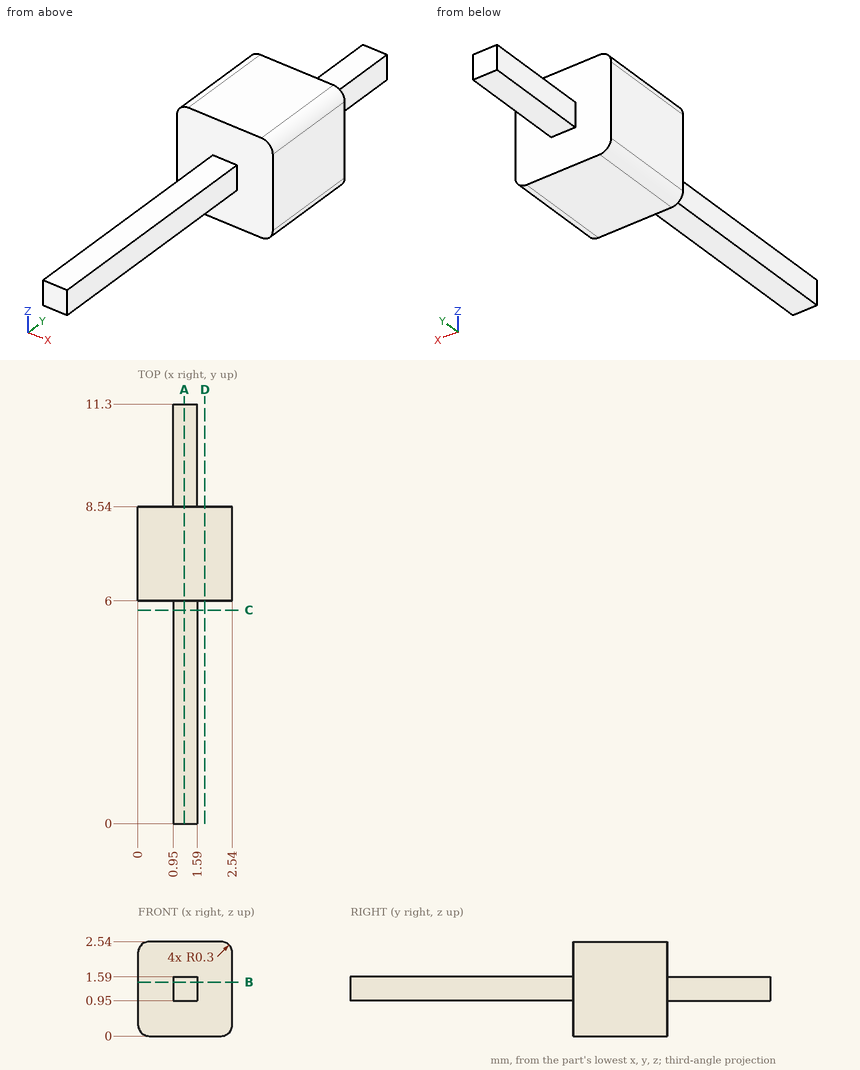
Input: dimensioned drawing with shaded views. Units: mm. Origin: part minimum x, y, z. Round coordinates to 2 decimals unless told otherwise and drop trailing zeros. Loops run counter-clockwise (first coordinate to the right, second up) from the corner with the lowest first, then second, coordinate; pieces in that order, holes last. Notation, with made-up numbers: M 66.5,-34 L 87.5,-34 A20 cw 87.5,-5 Z; hole C 45,43 d4. An arc over 180 degrees is marked long. Return JSON: item names as keys, results as strings. Group by question number.
1. Material intervals for line 1 along Y through (x, z) = (0.15, 0.2); line 2 along X through (y, z) = (6.5, 2.45), sorted ascending. Write a range as from..to.
2. Section query C-C on y = 5.75. Output: boundary loops of the cut face in (x, z), and give its area (3 significant figures).
3. Pin query (flat end, axial travel): pin 1 (0.5 mm diameter, centred on y = 10, z = 1.5, fed in from -X); pin 2 (0.7 mm diameter, centred on y = 10, z = 1, fed in from +X); pin 3 (1.3 mm diameter, centred on x = 1, z = 1.5, fed in from -Y). Return the tip coordinate at first contact, or that it passes through.
4. Section query B-B on z = 1.45. Output: boundary loops of the cut face in (x, y), and give its area (3 significant figures).
5. Section query A-A on x = 1.25. Output: boundary loops of the cut face in (y, z), and give its area (3 significant figures).
6. Section query D-D on x = 1.8. Output: boundary loops of the cut face in (y, z).
Checks:
{
 "1": {"line 1": "y = 6..8.54", "line 2": "x = 0.09..2.45"},
 "2": {"outline": "M 0.95,0.95 L 1.59,0.95 L 1.59,1.59 L 0.95,1.59 Z", "area": "0.410 mm²"},
 "3": {"pin 1": "stops at x = 0.95", "pin 2": "stops at x = 1.59", "pin 3": "stops at y = 0"},
 "4": {"outline": "M 0,6 L 0.95,6 L 0.95,0 L 1.59,0 L 1.59,6 L 2.54,6 L 2.54,8.54 L 1.59,8.54 L 1.59,11.3 L 0.95,11.3 L 0.95,8.54 L 0,8.54 Z", "area": "12.1 mm²"},
 "5": {"outline": "M 0,0.95 L 6,0.95 L 6,0 L 8.54,0 L 8.54,0.95 L 11.3,0.95 L 11.3,1.59 L 8.54,1.59 L 8.54,2.54 L 6,2.54 L 6,1.59 L 0,1.59 Z", "area": "12.1 mm²"},
 "6": {"outline": "M 6,0 L 8.54,0 L 8.54,2.54 L 6,2.54 Z"}
}
